Could you check a few things on this drawing? It's one solid part, dimensions in mm from its lowest x, y, z. Give positions to 0.01 mm unless a question says otherwise; leave off trailing zeros. Loops run counter-clockwise (first coordinate to the right, second up) from the corner with the lowest first, then second, coordinate; pieces in that order, holes last. Notation, with made-up numbers: (53.25, -18.75) - (96.25, -18.75) arc R10 ccw to (96.25, -4.75) - close; hole circle Ø4 at (6, -28.75). An arc over 180 degrees is marked (long way). Answer as a JSON object with one key per item and string values.
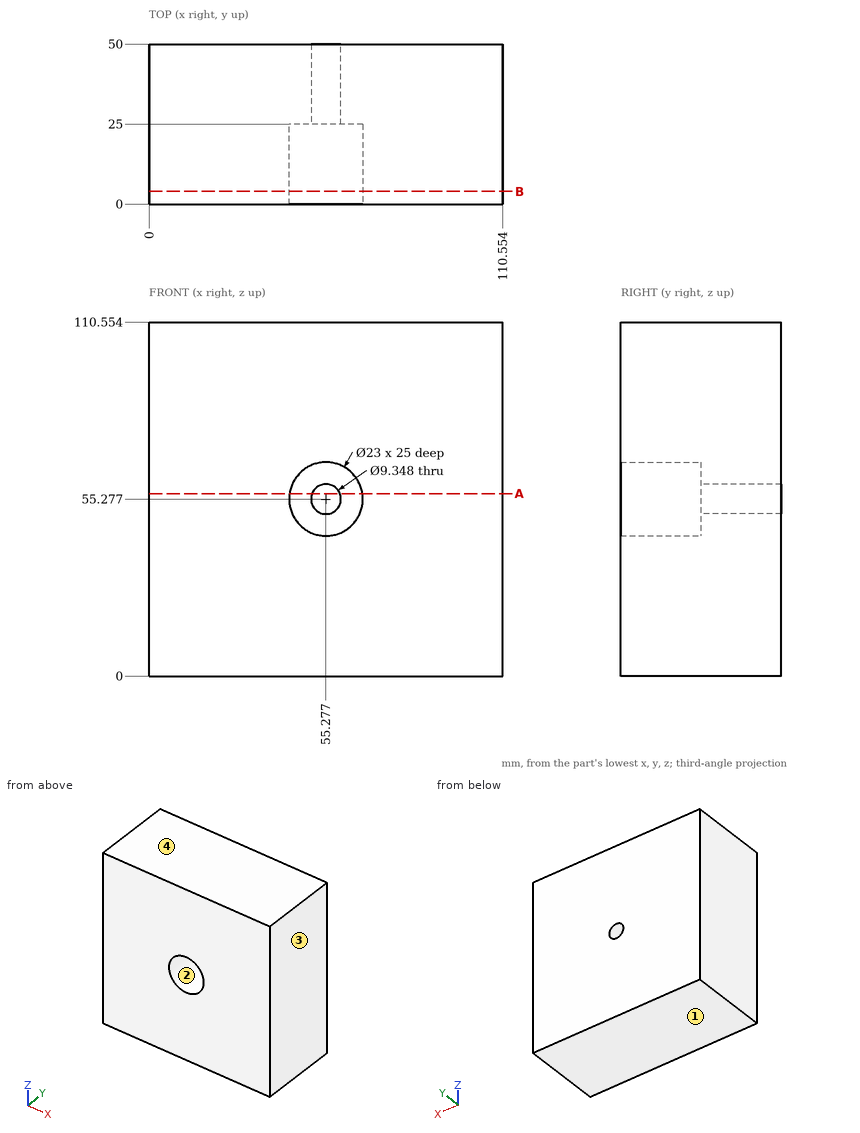
1) If we mould it in two halves opening along Z, with no side actions, what happens to the marked faces 1, 2, 3 and 4? For each: released by +Z, released by -Z, zero draft, split by the parting line, or undercut.
Check sheet entries:
{"face 1": "released by -Z", "face 2": "undercut", "face 3": "zero draft", "face 4": "released by +Z"}
2) I'm going to push flat-ended pins straight in: P1, Ø5.5, axis at x = 55.28, z = 55.28, coming from the -Y side; P2, Ø14, axis at x = 55.28, z = 55.28, coming from the -Y side. Where does each tip first touch, or does it pass through?
Check sheet entries:
{"P1": "through", "P2": "y = 25"}
3) I need wall thicknesses on L1, parallel to Y at x = 58.5, z = 50.5; L2, parallel to Z at x = 52.5, y = 8. Which ranges of each line are inside material? Lowest first, please.
Check sheet entries:
{"L1": "25 to 50", "L2": "0 to 44.12, 66.44 to 110.55"}
4) Imagine slicing it at B-B on y = 4. Write out the boundary of the cut face in (x, z), and give its area (3 significant figures).
Check sheet entries:
{"outline": "(0, 0) - (110.55, 0) - (110.55, 110.55) - (0, 110.55) - close; hole circle Ø23 at (55.28, 55.28)", "area": "11,800 mm2"}
5) Imagine slicing it at A-A on z = 57. Write out the boundary of the cut face in (x, y).
Check sheet entries:
{"outline": "(0, 0) - (43.91, 0) - (43.91, 25) - (50.93, 25) - (50.93, 50) - (0, 50) - close; (59.62, 25) - (66.65, 25) - (66.65, 0) - (110.55, 0) - (110.55, 50) - (59.62, 50) - close"}
